from build123d import *

# Parameters (mm, degrees)
SKETCH049_W             = 40
SKETCH049_H             = 15
PAD018_DEPTH            = 79
SKETCH050_W             = 40
SKETCH050_H             = 15
POCKET029_DEPTH         = 29
SKETCH051_W             = 40
SKETCH051_H             = 24
PAD019_DEPTH            = 40
SKETCH052_W             = 32
SKETCH052_H             = 16
POCKET030_DEPTH         = 40.001
FILLET008_R             = 3
BODY007_PLACEMENT_ANGLE = 90


with BuildPart() as part:
    # Sketch049 → Pad018 (new body)
    with BuildSketch(Plane.YZ):
        with Locations((20, 7.5)):
            Rectangle(SKETCH049_W, SKETCH049_H)
    extrude(amount=PAD018_DEPTH)

    # Sketch050 → Pocket029 (cut)
    with BuildSketch(Plane.YZ):
        with Locations((20, 7.5)):
            Rectangle(SKETCH050_W, SKETCH050_H)
        Polygon((3.5, 7.5), (7.5, 11.5), (33.5, 11.5), (37.5, 7.5), (33.5, 3.5), (7.5, 3.5), align=None, mode=Mode.SUBTRACT)
    extrude(amount=POCKET029_DEPTH, mode=Mode.SUBTRACT)

    # Sketch051 → Pad019 (join)
    with BuildSketch(Plane.XZ):
        with Locations((59, -12)):
            Rectangle(SKETCH051_W, SKETCH051_H)
    extrude(amount=-PAD019_DEPTH)

    # Sketch052 → Pocket030 (cut, through all)
    with BuildSketch(Plane.XZ):
        with Locations((55, -8)):
            Rectangle(SKETCH052_W, SKETCH052_H)
    extrude(amount=-POCKET030_DEPTH, mode=Mode.SUBTRACT)

    # Fillet008
    fillet008_edges = [part.edges().sort_by_distance(p)[0] for p in [
        (59, 40, -24),
        (39, 20, -24),
        (59, 0, -24),
        (39, 0, -20),
        (39, 40, -20),
        (39, 20, -16),
        (55, 0, -16),
        (55, 40, -16),
    ]]
    fillet(fillet008_edges, radius=FILLET008_R)


with BuildPart() as part_1:
    # Body007 placement: moved
    add(part.part.moved(Location((49.711133, -57.1, 20.293142))).rotate(Axis((49.711133, -57.1, 20.293142), (-1, 0, 0)), BODY007_PLACEMENT_ANGLE))


solid = part_1.part
Input: part model. Units: mm. Frame: model coordinates. A direction names the side the tool comes from. Coordinates: 2 decimals unless noted, no trailing zeros. Order: outer loops, then holes, each group sorted by start corner. A loop starts at its lowest first (then second) coordinate and runs counter-clockwise, first axis right, second up. Notation, with made-up numbers: M 32.25,-9 L 86.25,-9 A21 cw 86.25,-3 Z; hole C 21,-3.75 d8. An arc over 180 degrees is marked long. One line per question, with ' | ' between items.
Item 1: Reachability of faces 4 (the flat face through (64, -53.6, 0)), 5 (the cylindrical face through (89.567, -77.086, 19.391)), 6 (the flat face through (64.008, -47.628, 14.821)), 7 (the cylindrical face through (106.414, -73.955, 19.391)), 8 (the cylindrical face through (89.567, -77.086, -18.805)) from +Z, -Z, +X, -X, +Y, -Y: full face, straight path, thin tool, end or side. Return the list, or none.
Geometry results:
face 4: +Z, -Z, -X, -Y | face 5: +Z, -X, -Y | face 6: +Z, -X, +Y | face 7: +Z, -X | face 8: -Z, -X, -Y
Item 2: Section C-C (x = 58.5). Output: boundary loops of the cut face in (y, z).
Geometry results:
outline: M -53.6,-13.21 L -49.6,-17.21 L -45.6,-13.21 L -45.6,12.79 L -49.6,16.79 L -53.6,12.79 Z
Item 3: Pin query (flat end, axial travel): pin 1 (21 mm diameter, centred on y = -62, z = -1, fed in from -X); pin 2 (0.6 mm diameter, centred on y = -77.5, z = -4, fed in from -X); pin 3 (8 mm diameter, centred on x = 59.5, z = -6, fed in from +Y); pin 4 (21 mm diameter, centred on x = 58, z = 1.5, fed in from -Y). Return the tip coordinate at first contact, or that it passes through.
Geometry results:
pin 1: stops at x = 49.71 | pin 2: stops at x = 88.71 | pin 3: stops at y = -45.6 | pin 4: stops at y = -53.6
Item 4: Section D-D (y = -56). Output: boundary loops of the cut face in (x, z), then the cut area to 3 significant figures.
Geometry results:
outline: M 78.71,-19.71 L 128.71,-19.71 L 128.71,20.29 L 78.71,20.29 Z | area: 2,000 mm^2
Item 5: Ray query, line 1 along Y through (x, z) = (93, -1); line 2 along X through (y, z) = (-69.5, -14); line 3 along Y through (x, z) = (87, -15). Return the intervals inside material, ascending.
Geometry results:
line 1: y = -81.1 to -73.1, -57.1 to -42.1 | line 2: x = 120.71 to 128.71 | line 3: y = -57.1 to -42.1
Item 6: Draft query along Y for faces 1 (the cylindrical face through (106.41, -74, -18.85)), 2 (the flat face through (64, -45.6, 0)), 3 (the flat face through (49.711, -50, 0)). Return one class per face: released by +Y, released by -Y, zero draft, split by the parting line, or undercut.
Geometry results:
face 1: undercut | face 2: released by +Y | face 3: zero draft
Item 7: Section A-A (x = 94.5). Output: boundary loops of the cut face in (y, z).
Geometry results:
outline: M -81.1,-16.71 A3 ccw -78.1,-19.71 L -76.1,-19.71 A3 ccw -73.1,-16.71 L -73.1,17.29 A3 ccw -76.1,20.29 L -78.1,20.29 A3 ccw -81.1,17.29 Z; M -57.1,-19.71 L -42.1,-19.71 L -42.1,20.29 L -57.1,20.29 Z
Item 8: Section B-B (z = 9). Output: boundary loops of the cut face in (x, y).
Geometry results:
outline: M 49.71,-53.6 L 78.71,-53.6 L 78.71,-57.1 L 120.71,-57.1 L 120.71,-73.1 L 91.71,-73.1 A3 ccw 88.71,-76.1 L 88.71,-78.1 A3 ccw 91.71,-81.1 L 128.71,-81.1 L 128.71,-42.1 L 78.71,-42.1 L 78.71,-45.6 L 49.71,-45.6 Z
